Source: three-view drawing plus pictorial views. Frame: mm from the lowest corner of the part. Give positions to 0.01 mm unless a question says otherwise; leave off trailing zeros. Order: outer loops, then holes, each group sorted by start corner. A loop starts at its lowest first (then second) coordinate and runs counter-clockwise, first axis right, second up.
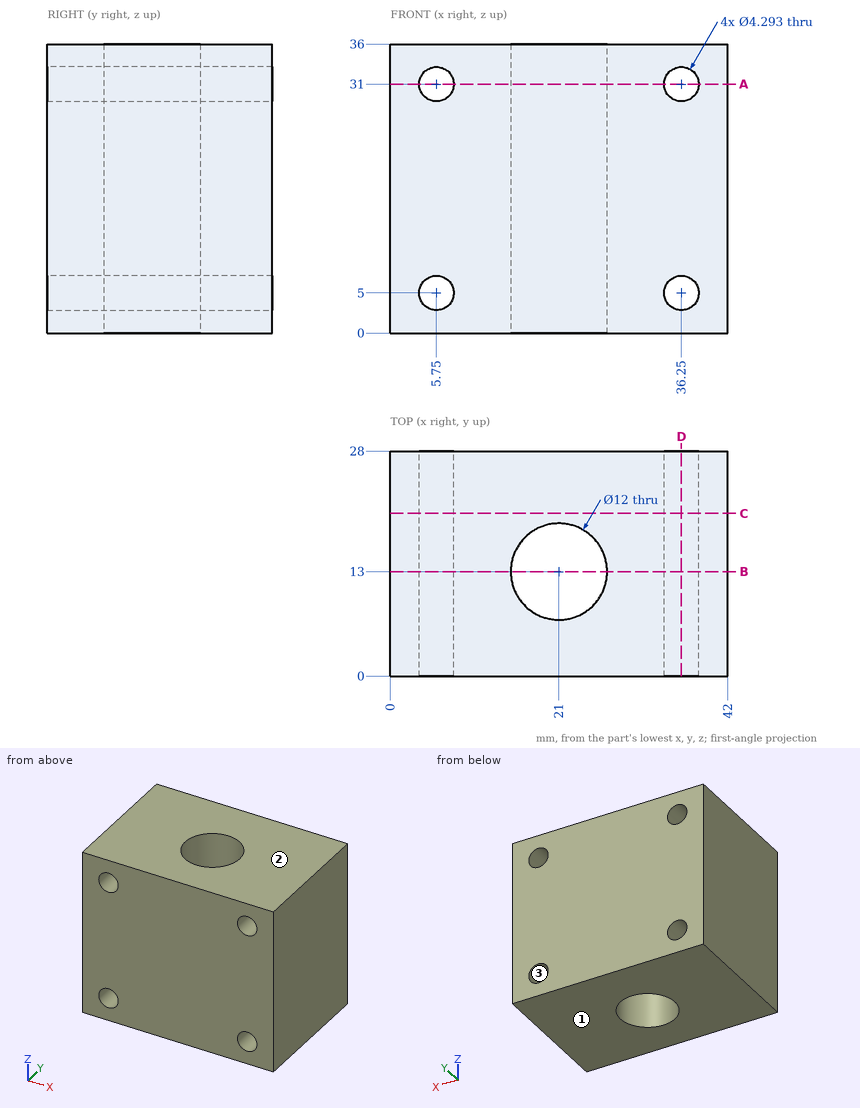
(1) Section D-D, the plane x = 36.25. Return loops of the section in (y, z).
(2) Section B-B, the plane y = 13. Return loops of the section in (x, z).
(3) Line query: line 1 along X through (y, z) = (19.25, 31); line 2 along Y through (x, z) = (21, 17.5); line 3 along X through (y, z) = (7.5, 31) (1 decimal). Output: solid intervals per line, ascending.
(4) Section C-C, the plane y = 20.25. Return loops of the section in (x, z), plus the area to 3 significant figures.
(5) Pin query (flat end, axial travel): pin 1 Ø2.5 at (x, z) = (5.75, 5) entering from -Y. Return the tip coordinate at first contact, or that it passes through.
(6) Section A-A, the plane z = 31. Return loops of the section in (x, y).
(7) Draft query along Z for the marked faces 1, 2 and 3. Return one class per face: +Z half, -Z half, draft (parallel to the pull), parting line (faces both ways), or undercut.
Checks:
1. outline: (0, 0) - (28, 0) - (28, 2.85) - (0, 2.85) - close; (0, 7.15) - (28, 7.15) - (28, 28.85) - (0, 28.85) - close; (0, 33.15) - (28, 33.15) - (28, 36) - (0, 36) - close
2. outline: (0, 0) - (15, 0) - (15, 36) - (0, 36) - close; (27, 0) - (42, 0) - (42, 36) - (27, 36) - close; hole circle Ø4.29 at (5.75, 5); hole circle Ø4.29 at (5.75, 31); hole circle Ø4.29 at (36.25, 5); hole circle Ø4.29 at (36.25, 31)
3. line 1: x = 0 to 3.6, 7.9 to 34.1, 38.4 to 42
3. line 2: y = 0 to 7, 19 to 28
3. line 3: x = 0 to 3.6, 7.9 to 18.6, 23.4 to 34.1, 38.4 to 42
4. outline: (0, 0) - (42, 0) - (42, 36) - (0, 36) - close; hole circle Ø4.29 at (5.75, 5); hole circle Ø4.29 at (5.75, 31); hole circle Ø4.29 at (36.25, 5); hole circle Ø4.29 at (36.25, 31)
4. area: 1,450 mm2
5. pin 1: passes through
6. outline: (0, 0) - (3.6, 0) - (3.6, 28) - (0, 28) - close; (7.9, 0) - (34.1, 0) - (34.1, 28) - (7.9, 28) - close; (38.4, 0) - (42, 0) - (42, 28) - (38.4, 28) - close; hole circle Ø12 at (21, 13)
7. face 1: -Z half
7. face 2: +Z half
7. face 3: undercut
